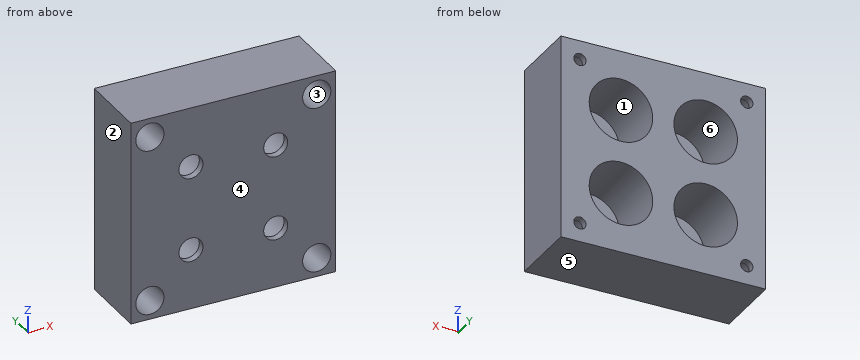
from build123d import *

# Parameters (mm, degrees)
SKETCH1_W           = 36.83
SKETCH1_H           = 36.83
SKETCH1_R           = 1.0999978
SKETCH1_R_2         = 2.159
BOSS_EXTRUDE1_DEPTH = 12.7
SKETCH2_R           = 5.715
CUT_EXTRUDE1_DEPTH  = 11.43
SKETCH3_R           = 2.54
CUT_EXTRUDE2_DEPTH  = 11.43


with BuildPart() as part:
    # Sketch1 → Boss-Extrude1 (new body)
    with BuildSketch(Plane(origin=(0, 0, 0), x_dir=(1, 0, 0), z_dir=(0, 1, 0))):
        with Locations((-1.422532637, -3.27613577)):
            Rectangle(SKETCH1_W, SKETCH1_H)
        with Locations(Location((-16.422528037, 11.72385963, 0), (0, 0, 270))):
            Circle(SKETCH1_R, mode=Mode.SUBTRACT)
        with Locations(Location((13.577462763, 11.72385963, 0), (0, 0, 90))):
            Circle(SKETCH1_R, mode=Mode.SUBTRACT)
        with Locations(Location((13.577462763, -18.27613117, 0), (0, 0, 270))):
            Circle(SKETCH1_R, mode=Mode.SUBTRACT)
        with Locations(Location((-16.422528037, -18.27613117, 0), (0, 0, 90))):
            Circle(SKETCH1_R, mode=Mode.SUBTRACT)
        with Locations(Location((-9.042532637, 4.34386423, 0), (0, 0, 270))):
            Circle(SKETCH1_R_2, mode=Mode.SUBTRACT)
        with Locations(Location((6.197467363, 4.34386423, 0), (0, 0, 90))):
            Circle(SKETCH1_R_2, mode=Mode.SUBTRACT)
        with Locations(Location((6.197467363, -10.89613577, 0), (0, 0, 270))):
            Circle(SKETCH1_R_2, mode=Mode.SUBTRACT)
        with Locations(Location((-9.042532637, -10.89613577, 0), (0, 0, 90))):
            Circle(SKETCH1_R_2, mode=Mode.SUBTRACT)
    extrude(amount=BOSS_EXTRUDE1_DEPTH)

    # Sketch2 → Cut-Extrude1 (cut)
    with BuildSketch(Plane(origin=(0, 12.7, 0), x_dir=(1, 0, 0), z_dir=(0, 1, 0))):
        with Locations(Location((-9.042532637, 4.34386423, 0), (0, 0, 270))):
            Circle(SKETCH2_R)
        with Locations(Location((6.197467363, 4.34386423, 0), (0, 0, 90))):
            Circle(SKETCH2_R)
        with Locations(Location((6.197467363, -10.89613577, 0), (0, 0, 270))):
            Circle(SKETCH2_R)
        with Locations(Location((-9.042532637, -10.89613577, 0), (0, 0, 90))):
            Circle(SKETCH2_R)
    extrude(amount=-CUT_EXTRUDE1_DEPTH, mode=Mode.SUBTRACT)

    # Sketch3 → Cut-Extrude2 (cut)
    with BuildSketch(Plane.XZ):
        with Locations(Location((-16.422528037, 18.27613117, 0), (0, 0, 270))):
            Circle(SKETCH3_R)
        with Locations(Location((13.577462763, 18.27613117, 0), (0, 0, 90))):
            Circle(SKETCH3_R)
        with Locations(Location((13.577462763, -11.72385963, 0), (0, 0, 270))):
            Circle(SKETCH3_R)
        with Locations(Location((-16.422528037, -11.72385963, 0), (0, 0, 90))):
            Circle(SKETCH3_R)
    extrude(amount=-CUT_EXTRUDE2_DEPTH, mode=Mode.SUBTRACT)


solid = part.part
The listing builds one solid part. Answer for the finished solid, in the listing's coordinates (mm). Face numbers are marked on the shaded views. A direction names the side the tool comes from. Coordinates: 2 decimals unless noted, no trailing zeros. Write each loop counter-clockwise with the first axis right and the second up, starting at its lowest first coordinate (ties: lowest second). Pieces come first, ordered by that corner, then holes. Notation, with made-up numbers: (44.5, 44) - (97.5, 44) arc R16 cw to (97.5, 66) - close; hole circle Ø3 at (61, 8). An arc over 180 degrees is marked (long way). Return JSON: item names as keys, results as strings.
1. The part is cut by section C-C on y = 7.5. Count the separate pieces of the cut face and the enclosed holes in it, then the cut area to 3 significant figures.
Final values:
{"separate pieces": "1", "enclosed holes": "8", "area": "865 mm^2"}
2. Which of the six approach directions +Z, -Z, +X, -X, +Y, -Y give full straight-line access (tool end or side, diameter ignored) to the marked faces 1, 2 and 3?
Final values:
{"face 1": "+Y", "face 2": "+Z, -Z, -X, +Y, -Y", "face 3": "-Y"}
3. Consider line 1 along Z through (x, y) = (6, 8.25); line 2 along Z through (x, y) = (-11.5, 8.25); line 3 along X through (y, z) = (4, 19). Determine where each line is inside the solid, lowest interval first.
Final values:
{"line 1": "-15.14 to -10.06, 1.37 to 5.18, 16.61 to 21.69", "line 2": "-15.14 to -9.5, 0.82 to 5.74, 16.06 to 21.69", "line 3": "-19.84 to -18.86, -13.99 to 11.14, 16.01 to 16.99"}
4. For a pull along Z with two mould halves and no side action, classify the marked faces 4, 5 and 6 as +Z half, -Z half, draft (parallel to the pull), parting line (faces both ways), or undercut.
Final values:
{"face 4": "draft", "face 5": "-Z half", "face 6": "undercut"}
5. The part is cut by section D-D on x = 9.5. Determine the outline of the cut face in (y, z), then the cut area to 3 significant figures.
Final values:
{"outline": "(0, -15.14) - (12.7, -15.14) - (12.7, -9.01) - (1.27, -9.01) - (1.27, 0.32) - (12.7, 0.32) - (12.7, 6.23) - (1.27, 6.23) - (1.27, 15.56) - (12.7, 15.56) - (12.7, 21.69) - (0, 21.69) - close", "area": "254 mm^2"}
6. The part is cut by section A-A on z = -12. Determine the outline of the cut face in (x, y), then the cut area to 3 significant figures.
Final values:
{"outline": "(-19.84, 0) - (-18.95, 0) - (-18.95, 11.43) - (-17.49, 11.43) - (-17.49, 12.7) - (-19.84, 12.7) - close; (-15.36, 11.43) - (-13.9, 11.43) - (-13.9, 0) - (11.05, 0) - (11.05, 11.43) - (12.51, 11.43) - (12.51, 12.7) - (-15.36, 12.7) - close; (14.64, 11.43) - (16.1, 11.43) - (16.1, 0) - (16.99, 0) - (16.99, 12.7) - (14.64, 12.7) - close", "area": "347 mm^2"}
7. The part is cut by section B-B on x = 5.5. Determine the outline of the cut face in (y, z).
Final values:
{"outline": "(0, -15.14) - (12.7, -15.14) - (12.7, -10.02) - (1.27, -10.02) - (1.27, -6.39) - (0, -6.39) - close; (0, -2.3) - (1.27, -2.3) - (1.27, 1.33) - (12.7, 1.33) - (12.7, 5.22) - (1.27, 5.22) - (1.27, 8.85) - (0, 8.85) - close; (0, 12.94) - (1.27, 12.94) - (1.27, 16.57) - (12.7, 16.57) - (12.7, 21.69) - (0, 21.69) - close"}
8. Each of these flat-tipped pins is pushed along its axis until it touches: pin 1 Ø7 at (x, z) = (6.2, -4.34) entering from +Y; pin 2 Ø1.3 at (x, z) = (13.58, -11.72) entering from -Y. Where does it stop, or does it pass through?
Final values:
{"pin 1": "y = 1.27", "pin 2": "through"}
